Here's how the part is built. I have some questions about the finished solid (model axes, mm). A direction names the side the tool comes from. Give positions to 0.01 mm unless a question says otherwise; leave off trailing zeros. Loops run counter-clockwise (first coordinate to the right, second up) from the corner with the lowest first, then second, coordinate; pieces in that order, holes last. Notation, with made-up numbers: (-37, 13) - (-5, 13) arc R23 cw to (-5, 51) - close; hole circle Ø10 at (-34, 72.5). An arc over 180 degrees is marked (long way). Use a Markdown table: item, result.
Autodesk Inventor part; units mm, degrees
ref_plane "YZ Plane" through (0, 0, 0) normal (1, 0, 0) x (0, 1, 0)
ref_plane "XZ Plane" through (0, 0, 0) normal (0, 1, 0) x (-1, 0, 0)
ref_plane "XY Plane" through (0, 0, 0) normal (0, 0, 1) x (1, 0, 0)
sketch "Sketch1" plane through (0, 0, 0) normal (0, 1, 0) x (-1, 0, 0)
  line L0 (0, 0) -> (70, 0)
  line L1 (70, 0) -> (70, -50)
  line L2 (70, -50) -> (0, -50)
  line L3 (0, -50) -> (0, 0)
  dimension "d0" = 70
  dimension "d1" = 50
extrude "Extrusion1" add sketch "Sketch1" along normal blind 6
sketch "Sketch2" plane through (0, 6, 0) normal (0, 1, 0) x (1, 0, 0)
  circle A0 centre (-11, 11) radius 2.75
  line L0 (0, 0) -> (0, 50)
  line L1 (-70, 0) -> (0, 0)
  dimension "d4" = 5.5
  dimension "d5" = 11
  dimension "d6" = 11
extrude "Extrusion2" cut sketch "Sketch2" against normal through all
pattern_linear "Rectangular Pattern1" count 2 spacing 38 along (-1, 0, 0) count 2 spacing 25 along (0, 0, -1) of "Extrusion2"
sketch "Sketch3" plane through (0, 6, 0) normal (0, 1, 0) x (1, 0, 0)
  circle A0 centre (-49, 11) radius 2.75
  line L0 (-49, 11) -> (-59, 11) construction
  line L1 (-49, 13.75) -> (-59, 13.75)
  line L2 (-59, 8.25) -> (-49, 8.25)
  arc A1 (-49, 8.25) -> (-49, 13.75) centre (-49, 11) ccw
  arc A2 (-59, 13.75) -> (-59, 8.25) centre (-59, 11) ccw
  circle A3 centre (-49, 36) radius 2.75
  line L3 (-49, 36) -> (-59, 36) construction
  line L4 (-49, 38.75) -> (-59, 38.75)
  line L5 (-59, 33.25) -> (-49, 33.25)
  arc A4 (-49, 33.25) -> (-49, 38.75) centre (-49, 36) ccw
  arc A5 (-59, 38.75) -> (-59, 33.25) centre (-59, 36) ccw
  point P0 (0, 0)
  point P1 (-54, 11)
  point P2 (-54, 36)
  dimension "d15" = 10
  dimension "d16" = 5.5
  dimension "d17" = 10
  dimension "d18" = 5.5
extrude "Extrusion3" cut sketch "Sketch3" against normal through all
properties part number "Y_Carriage_Plate"
(1) If I drill on line 1 (Z direction, x = -11, y = 4.7); line 2 (X direction, y = 4.85, z = -36); line 3 (X direction, y = 3.3, z = -34.5), over which ranges is the centre line in solid material (lowest first)?
A:
| item | result |
|---|---|
| line 1 | -50 to -38.75, -33.25 to -13.75, -8.25 to 0 |
| line 2 | -70 to -61.75, -46.25 to -13.75, -8.25 to 0 |
| line 3 | -70 to -61.3, -46.7 to -13.3, -8.7 to 0 |
(2) Suppose I cut it at C-C on y = 1.9. Write out the boundary of the cut face in (x, z), plus the area to 3 significant figures.
A:
| item | result |
|---|---|
| outline | (-70, -50) - (0, -50) - (0, 0) - (-70, 0) - close; hole (-59, -38.75) - (-49, -38.75) arc R2.75 ccw to (-49, -33.25) - (-59, -33.25) arc R2.75 ccw to start; hole (-59, -13.75) - (-49, -13.75) arc R2.75 ccw to (-49, -8.25) - (-59, -8.25) arc R2.75 ccw to start; hole circle Ø5.5 at (-11, -36); hole circle Ø5.5 at (-11, -11) |
| area | 3,290 mm2 |
(3) On a 3-axis mill with a long thin cutter (end or side, diameter ignored), from which of +Z, -Z, +X, -X, +Y, -Y can I reach the whole of each face in a straight line? I mean faces 1 (the face through (-61.75, 3.04, -11.06)), 2 (the face through (-35, 6, -25)). Say none if no direction works.
A:
| item | result |
|---|---|
| face 1 | +Y, -Y |
| face 2 | +Z, -Z, +X, -X, +Y |
(4) We'd pull the mould along X, two halves only. Please class faces 3 (the face through (0, 3, -25)), 4 (the face through (-35, 3, -50)), 5 (the face through (-54, 3, -33.25)): pulls with the +X half, pulls with the -X half, needs draft (parallel to the pull), parting line crosses it, or undercut.
A:
| item | result |
|---|---|
| face 3 | pulls with the +X half |
| face 4 | needs draft |
| face 5 | undercut |
(5) Suppose I cut it at A-A on x = -11. Write out the boundary of the cut face in (y, z).
A:
| item | result |
|---|---|
| outline | (0, -50) - (6, -50) - (6, -38.75) - (0, -38.75) - close; (0, -33.25) - (6, -33.25) - (6, -13.75) - (0, -13.75) - close; (0, -8.25) - (6, -8.25) - (6, 0) - (0, 0) - close |
(6) Suppose I cut it at B-B on z = -11. Write out the boundary of the cut face in (x, y), plus the area to 3 significant figures.
A:
| item | result |
|---|---|
| outline | (-70, 0) - (-61.75, 0) - (-61.75, 6) - (-70, 6) - close; (-46.25, 0) - (-13.75, 0) - (-13.75, 6) - (-46.25, 6) - close; (-8.25, 0) - (0, 0) - (0, 6) - (-8.25, 6) - close |
| area | 294 mm2 |
(7) Will this pin go through, and if not, where does the flat tip stop? pin 1 (6 mm diameter, centred on x = -45, z = -5, fed in from -Y).
A:
| item | result |
|---|---|
| pin 1 | y = 0 |
